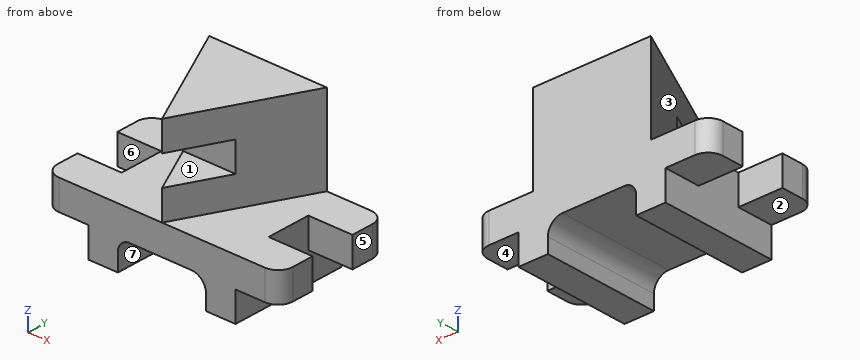
```python
from build123d import *

# Parameters (mm, degrees)
F0_W      = 203.2
F0_H      = 25.4
F1_DEPTH  = 50.8
F3_DEPTH  = 25.4
F5_DEPTH  = 50.8
F7_DEPTH  = 25.4
F8_W      = 38.1
F8_H      = 38.1
F9_DEPTH  = 25.401
F10_R     = 12.7
F11_W     = 127
F11_H     = 25.4
F12_DEPTH = 101.6
F13_W     = 76.2
F13_H     = 25.4
F14_DEPTH = 101.601
F15_R     = 10.16
F16_R     = 12.7


with BuildPart() as f1:
    # F0 (on Front) → F1 (new body, symmetric)
    with BuildSketch(Plane.XZ):
        with Locations((101.6, 12.7)):
            Rectangle(F0_W, F0_H)
    extrude(amount=F1_DEPTH, both=True)

    # F2 (on face) → F3 (join)
    with BuildSketch(Plane.XY.offset(25.4)):
        Polygon((50.8, 50.8), (101.6, -50.8), (152.4, 50.8), align=None)
    extrude(amount=F3_DEPTH)

    # F4 (on face) → F5 (join)
    with BuildSketch(Plane.XY.offset(50.8)):
        Polygon((50.8, 50.8), (78.8815493486, -5.3630986972), (124.3184506514, -5.3630986972), (152.4, 50.8), align=None)
    extrude(amount=F5_DEPTH)

    # F6 (on face) → F7 (join)
    with BuildSketch(Plane.XY.offset(101.6)):
        Polygon((124.3184506514, -5.3630986972), (78.8815493486, -5.3630986972), (101.6, -50.8), align=None)
        Polygon((50.8, 50.8), (78.8815493486, -5.3630986972), (124.3184506514, -5.3630986972), (152.4, 50.8), align=None)
    extrude(amount=-F7_DEPTH)

    # F8 (on face) → F9 (cut, through all)
    with BuildSketch(Plane.XY.offset(25.4)):
        with Locations((19.05, 0)):
            Rectangle(F8_W, F8_H)
        with Locations((184.15, 0)):
            Rectangle(F8_W, F8_H)
    extrude(amount=-F9_DEPTH, mode=Mode.SUBTRACT)

    # F10
    f10_edges = [f1.edges().sort_by_distance(p)[0] for p in [
        (0, 50.8, 12.7),
        (0, -50.8, 12.7),
        (203.2, -50.8, 12.7),
        (203.2, 50.8, 12.7),
    ]]
    fillet(f10_edges, radius=F10_R)

    # F11 (on face) → F12 (join, through all)
    with BuildSketch(Plane.XZ.offset(50.8)):
        with Locations((101.6, -12.7)):
            Rectangle(F11_W, F11_H)
    extrude(amount=-F12_DEPTH)

    # F13 (on face) → F14 (cut, through all)
    with BuildSketch(Plane.XZ.offset(50.8)):
        with Locations((101.6, -12.7)):
            Rectangle(F13_W, F13_H)
    extrude(amount=-F14_DEPTH, mode=Mode.SUBTRACT)

    # F15
    f15_edges = [f1.edges().sort_by_distance(p)[0] for p in [
        (63.5, 0, 0),
    ]]
    fillet(f15_edges, radius=F15_R)

    # F16
    f16_edges = [f1.edges().sort_by_distance(p)[0] for p in [
        (139.7, 0, 0),
    ]]
    fillet(f16_edges, radius=F16_R)


solid = f1.part
```
Read the model definition and answer for the solid it produces. Units are mm, in the model's axes. Face numbers are marked on the shaded views. A direction names the side the tool comes from. Give positions to 0.01 mm unless a question says otherwise; leave off trailing zeros. Order: outer loops, then holes, each group sorted by start corner. A loop starts at its lowest first (then second) coordinate and runs counter-clockwise, first axis right, second up.
(1) Find section A-A (y = -34.5). Give the vertices of the cut face in (x, z).
(2) Find section C-C (z = -7.5). Give the vertices of the cut face in (x, y), plus the area to 3 significant figures.
(3) For the marked faces 1, 2, 3 and 4, determine the directions among +Z, -Z, +X, -X, +Y, -Y from which every point of the face is accessible in a straight line to the end or side of a thin tool.
(4) For a pull along X with two mould halves and no side action, classify the marked faces 5, 6 and 7 as released by +X, released by -X, zero draft, split by the parting line, or undercut.
(5) Straight lines are drawn through the part: L1, parallel to Y at x = 14, z = 25; L2, parallel to Z at x = 92, y = 9; L3, parallel to X at y = 17, z = 21. For each, find the intervals that lie inside material, in ascending order.
(6) Given pin 1 (7.5 mm diameter, centred on x = 94, z = 61, fed in from -Y); pin 2 (16 mm diameter, centred on x = 16, y = -28, fed in from -Z); pin 3 (10 mm diameter, centred on y = 25, z = -21, fed in from -X), each flat-ended and moving along its own axis, determine where each tip first touches the part or whether it passes through.
(7) Find section B-B (x = 176). Give the vertices of the cut face in (y, z), plus the area to 3 significant figures.
(8) Find section D-D (y = 11.5). Give the vertices of the cut face in (x, z).
Result sheet:
1. outline: (0, 0) - (38.1, 0) - (38.1, -25.4) - (63.5, -25.4) - (63.5, -10.16) arc R10.16 cw to (73.66, 0) - (127, 0) arc R12.7 cw to (139.7, -12.7) - (139.7, -25.4) - (165.1, -25.4) - (165.1, 0) - (203.2, 0) - (203.2, 25.4) - (109.75, 25.4) - (109.75, 50.8) - (93.45, 50.8) - (93.45, 25.4) - (0, 25.4) - close; (93.45, 76.2) - (109.75, 76.2) - (109.75, 101.6) - (93.45, 101.6) - close
2. outline: (38.1, -50.8) - (63.85, -50.8) - (63.85, 50.8) - (38.1, 50.8) - close; (138.59, -50.8) - (165.1, -50.8) - (165.1, 50.8) - (138.59, 50.8) - close
2. area: 5,310 mm2
3. face 1: +X, -X, -Y
3. face 2: -Z, -X, +Y, -Y
3. face 3: +Z, -X, -Y
3. face 4: -Z, +X, +Y, -Y
4. face 5: released by +X
4. face 6: zero draft
4. face 7: undercut
5. L1: y = -50.8 to -19.05, 19.05 to 50.8
5. L2: z = 0 to 101.6
5. L3: x = 38.1 to 165.1
6. pin 1: stops at y = -5.36
6. pin 2: stops at z = 0
6. pin 3: stops at x = 38.1
7. outline: (-50.8, 0) - (-19.05, 0) - (-19.05, 25.4) - (-50.8, 25.4) - close; (19.05, 0) - (50.8, 0) - (50.8, 25.4) - (19.05, 25.4) - close
7. area: 1,610 mm2
8. outline: (38.1, -25.4) - (63.5, -25.4) - (63.5, -10.16) arc R10.16 cw to (73.66, 0) - (127, 0) arc R12.7 cw to (139.7, -12.7) - (139.7, -25.4) - (165.1, -25.4) - (165.1, 25.4) - (132.75, 25.4) - (132.75, 101.6) - (70.45, 101.6) - (70.45, 25.4) - (38.1, 25.4) - close
